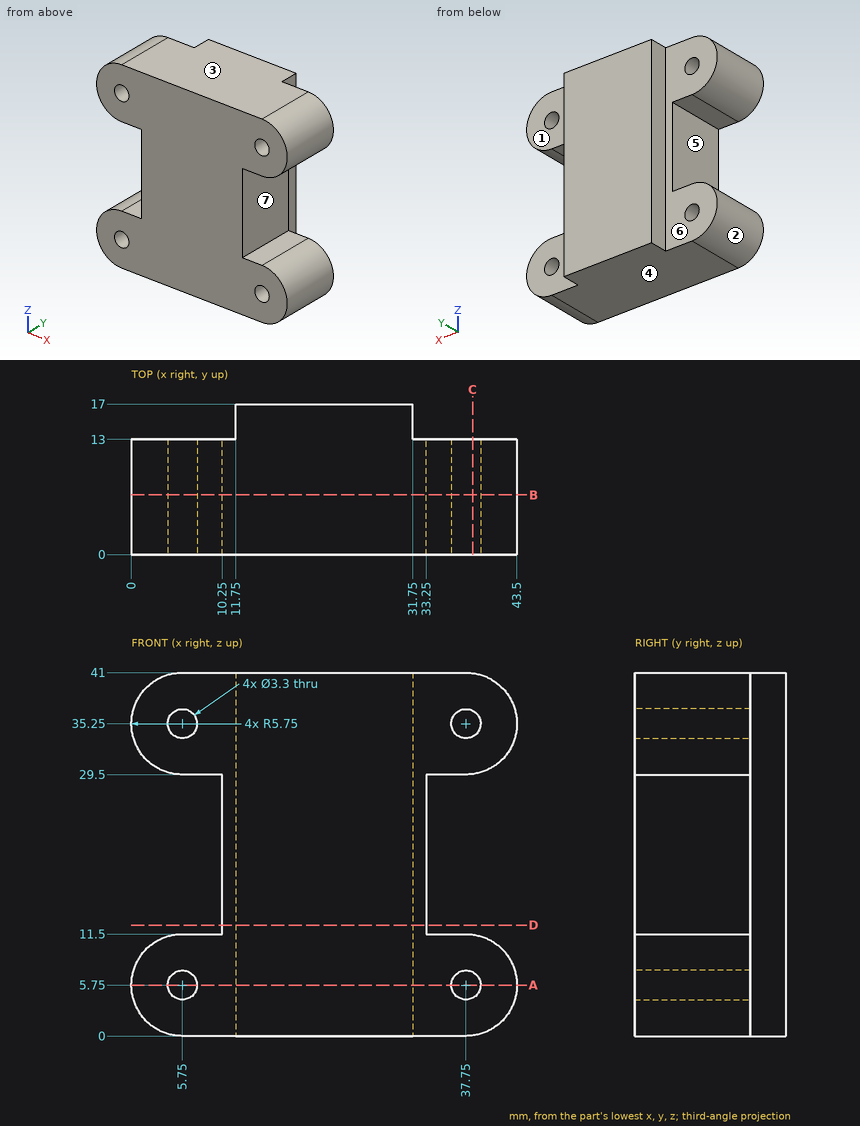
Verification items for this drawing (mm, ordinates from the low corner). A direction names the side the tool comes from. Round coordinates to 2 decimals unless told otherwise and drop trailing zeros. Loops run counter-clockwise (first coordinate to the right, second up) from the corner with the lowest first, then second, coordinate; pieces in that order, holes last. Notation, with made-up numbers: (35, 10) - (72, 10) arc R12 ccw to (72, 30) - close; hole circle Ø6 at (64, 17). An arc over 180 degrees is marked (long way). Write item = value, one per line.
Q1. Sectioned sample at C-C on x = 38.5. Record the boundary of the cut face in (y, z), plus the area to 3 significant figures.
Here are the results:
outline = (0, 0.05) - (13, 0.05) - (13, 4.28) - (0, 4.28) - close; (0, 7.22) - (13, 7.22) - (13, 11.45) - (0, 11.45) - close; (0, 29.55) - (13, 29.55) - (13, 33.78) - (0, 33.78) - close; (0, 36.72) - (13, 36.72) - (13, 40.95) - (0, 40.95) - close
area = 220 mm^2
Q2. Sectioned sample at A-A on z = 5.75. Record the boundary of the cut face in (x, y).
Here are the results:
outline = (0, 0) - (4.1, 0) - (4.1, 13) - (0, 13) - close; (7.4, 0) - (36.1, 0) - (36.1, 13) - (31.75, 13) - (31.75, 17) - (11.75, 17) - (11.75, 13) - (7.4, 13) - close; (39.4, 0) - (43.5, 0) - (43.5, 13) - (39.4, 13) - close
Q3. Depth check by flat-ended pin: pin 1 (4 mm diameter, centred on y = 8, z = 23, fed in from -X); pin 2 (5.5 mm diameter, centred on x = 5.75, z = 35.25, fed in from +Y); pin 3 (3 mm diameter, centred on y = 15.5, z = 22.5, fed in from -X); pin 4 (2 mm diameter, centred on x = 37.75, z = 5.75, fed in from -Y). Enter the tip coordinate at first touch or a pass-through.
Here are the results:
pin_1 = 10.25
pin_2 = 13
pin_3 = 11.75
pin_4 = through
Q4. Sectioned sample at B-B on y = 6.75. Record the boundary of the cut face in (x, z).
Here are the results:
outline = (5.75, 0) - (37.75, 0) arc R5.75 ccw to (37.75, 11.5) - (33.25, 11.5) - (33.25, 29.5) - (37.75, 29.5) arc R5.75 ccw to (37.75, 41) - (5.75, 41) arc R5.75 ccw to (5.75, 29.5) - (10.25, 29.5) - (10.25, 11.5) - (5.75, 11.5) arc R5.75 ccw to start; hole circle Ø3.3 at (5.75, 5.75); hole circle Ø3.3 at (5.75, 35.25); hole circle Ø3.3 at (37.75, 5.75); hole circle Ø3.3 at (37.75, 35.25)
Q5. Material ranges on L1, parallel to X at y = 9.25, z = 35.25; L2, parallel to Z at x = 37.75, y = 6.75; L3, parallel to Z at x = 35, y = 12.25, recorded low to high.
Here are the results:
L1 = 0 to 4.1, 7.4 to 36.1, 39.4 to 43.5
L2 = 0 to 4.1, 7.4 to 11.5, 29.5 to 33.6, 36.9 to 41
L3 = 0 to 11.5, 29.5 to 41
Q6. Mould release check, pull along Z, two halves, no side actions. Record for the marked faces 1, 2, 3 and 4: +Z half, -Z half, draft (parallel to the pull), parting line (faces both ways), or undercut.
Here are the results:
face_1 = draft
face_2 = undercut
face_3 = +Z half
face_4 = -Z half
Q7. Sectioned sample at D-D on z = 12.5. Record the boundary of the cut face in (x, y).
Here are the results:
outline = (10.25, 0) - (33.25, 0) - (33.25, 13) - (31.75, 13) - (31.75, 17) - (11.75, 17) - (11.75, 13) - (10.25, 13) - close
Q8. Tool access check on the marked faces 5, 6 and 7. Record the directions out of +Z, -Z, +X, -X, +Y, -Y that give a thin tool (end or side, any length) a straight path to the whole face; none if there is none.
Here are the results:
face_5 = -X, +Y, -Y
face_6 = +Z, -Z, -X, +Y
face_7 = +X, +Y, -Y
